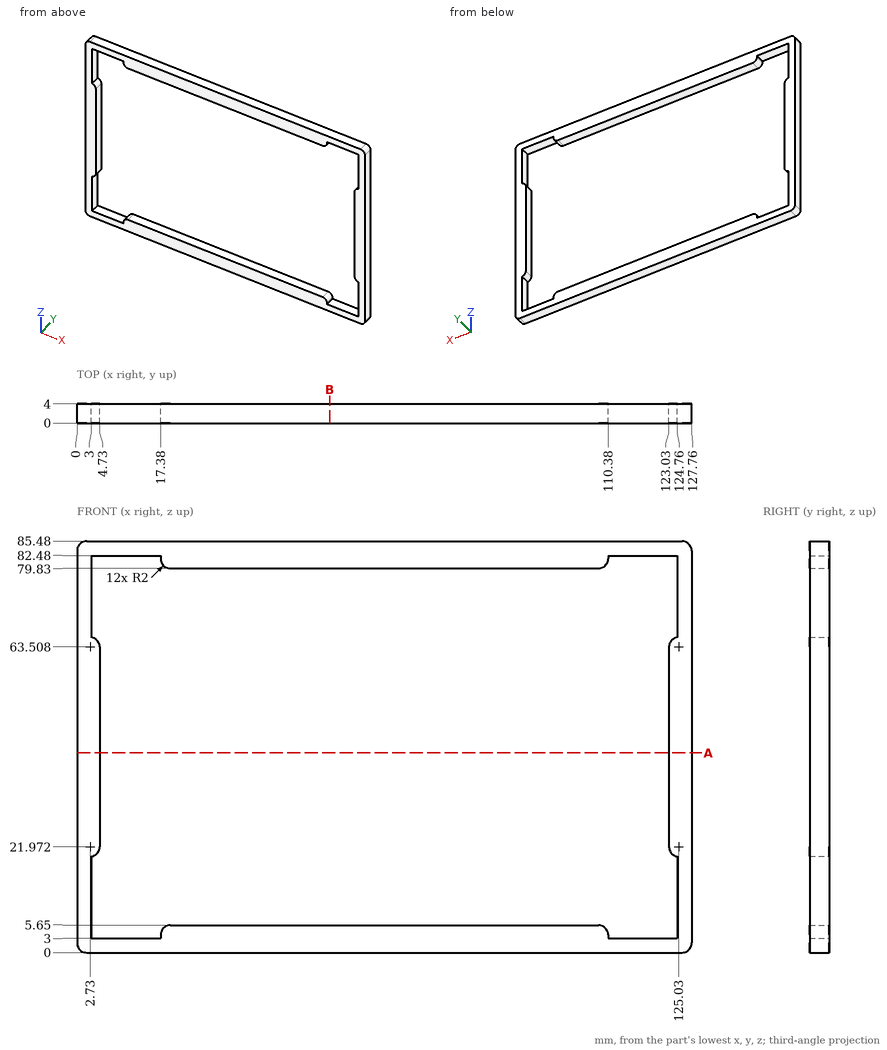
For this review, use the dimensioned drawing (mm, ordinates from the lowest corner) and the shaded views. Coordinates: 2 decimals unless noted, no trailing zeros. Order: outer loops, then holes, each group sorted by start corner. A loop starts at its lowest first (then second) coordinate and runs counter-clockwise, first axis right, second up. Notation, with made-up numbers: (66, 53) - (89, 53) arc R15 ccw to (89, 57) - close; hole circle Ø8 at (22, -34). An arc over 180 degrees is marked (long way). Use one line per item in the form item = value.
Q1. For P1, Ø12, axis at x = 70, z = 11, coming from the -Y side, flat-tipped, find the tip position at first contact; note if it passes through.
Checked values:
P1 = 0
Q2. Consider section A-A (z = 41.5). Give the boundary of the cut face in (x, y).
Checked values:
outline = (0, 0) - (4.73, 0) - (4.73, 4) - (0, 4) - close; (123.03, 0) - (127.76, 0) - (127.76, 4) - (123.03, 4) - close
Q3. For probe 1 along Z at (x, y) = (36, 2.3); probe 2 along Z at (x, y) = (121, 2.15); probe 3 along X at (y, z) = (2.1, 60.5), list the stretches that pass through material, from the lowest coordinate up. Write a range as from..to.
Checked values:
probe_1 = 0..5.65, 79.83..85.48
probe_2 = 0..3, 82.48..85.48
probe_3 = 0..4.73, 123.03..127.76
Q4. Consider section B-B (x = 52.5). Give the boundary of the cut face in (y, z), then the cut area to 3 significant figures.
Checked values:
outline = (0, 0) - (4, 0) - (4, 5.65) - (0, 5.65) - close; (0, 79.83) - (4, 79.83) - (4, 85.48) - (0, 85.48) - close
area = 45.2 mm2
